Input: part model. Units: mm. Frame: model coordinates. A direction names the side the tool comes from. Coordinates: 2 decimals unless noted, no trailing zeros. Write each loop counter-clockwise with the first axis right and the second up, starting at its lowest first coordinate (ties: lowest second). Pieces come first, ordered by that corner, then holes. Notation, with made-up numbers: (87, 67) - (126, 67) arc R21 ccw to (126, 86) - close; hole circle Ø3 at (-30.75, -23.5). An arc over 180 degrees is marked (long way). One line per question, with ' | ' between items. Start each with the question number.
1) First-contact query: P1, Ø1, axis at x = 2, y = -3.5, coming from the -Z side; P2, Ø1, axis at y = 4, z = -2.5, coming from the -X side; P3, Ø0.8, axis at x = -2.5, y = 3, coming from the -Z side. Flat tips, straight axial feed; report the tip coordinate or a pass-through.
2) Section query A-A on y = 0. Return loops of the section in (x, z), and give its area (3 significant figures).
3) Line query: line 1 (Y direction, x = 0, z = 0.9); line 2 (Z direction, x = -3.5, y = 0.5); line 3 (Y direction, x = -1.75, z = 0.2). Output: solid intervals per line, ascending.
4) Section query B-B on z = 0.65. Return loops of the section in (x, y), and give its area (3 significant figures).
5) Section query C-C on x = 1.5. Return loops of the section in (y, z), and give its area (3 significant figures).
6) Reachability of faces 1 (the flat face through (-2.5, -4.5, -0.5)), 2 (the cylindrical face through (-4.93, 4.94, 1.01)), 3 (the cylindrical face through (-2.565, 3.496, -0.246)) from +Z, -Z, +X, -X, +Y, -Y: full face, straight path, thin tool, end or side. Return the list, or none.
7) Section query D-D on y = 3. Return loops of the section in (x, z).
```python
from build123d import *

# Parameters (mm, degrees)
SKETCH3_W           = 11
SKETCH3_H           = 12.04
BOSS_EXTRUDE1_DEPTH = 2
FILLET1_R           = 2
SKETCH4_R           = 2
CUT_EXTRUDE1_DEPTH  = 2
SKETCH5_R           = 0.5
BOSS_EXTRUDE2_DEPTH = 0.5
SKETCH6_R           = 0.5
BOSS_EXTRUDE3_DEPTH = 4


with BuildPart() as part:
    # Sketch3 → Boss-Extrude1 (new body)
    with BuildSketch(Plane.XY):
        with Locations((0, -0.48)):
            Rectangle(SKETCH3_W, SKETCH3_H)
    extrude(amount=BOSS_EXTRUDE1_DEPTH)

    # Fillet1
    fillet1_edges = [part.edges().sort_by_distance(p)[0] for p in [
        (-5.5, 5.54, 1),
        (5.5, 5.54, 1),
    ]]
    fillet(fillet1_edges, radius=FILLET1_R)

    # Sketch4 → Cut-Extrude1 (cut)
    with BuildSketch(Plane.XY):
        Circle(SKETCH4_R)
    extrude(amount=CUT_EXTRUDE1_DEPTH, mode=Mode.SUBTRACT)

    # Sketch5 → Boss-Extrude2 (add)
    with BuildSketch(Plane.XY):
        with Locations((2.5, 3)):
            Circle(SKETCH5_R)
        with Locations((-2.5, 3)):
            Circle(SKETCH5_R)
        with Locations((2.5, -4.493)):
            Circle(SKETCH5_R)
        with Locations((-2.5, -4.493)):
            Circle(SKETCH5_R)
    extrude(amount=-BOSS_EXTRUDE2_DEPTH)

    # Sketch6 → Boss-Extrude3 (add)
    with BuildSketch(Plane(origin=(0, 0, 0), x_dir=(-1, 0, 0), z_dir=(0, 0, -1))):
        with Locations(Location((0, -6, 0), (0, 0, 270))):
            Circle(SKETCH6_R)
        with Locations(Location((2.5, -6, 0), (0, 0, 270))):
            Circle(SKETCH6_R)
        with Locations(Location((-2.5, -6, 0), (0, 0, 270))):
            Circle(SKETCH6_R)
    extrude(amount=BOSS_EXTRUDE3_DEPTH)


solid = part.part
```
Answer key:
1) P1: z = 0 | P2: through | P3: z = -0.5
2) outline: (-5.5, 0) - (-2, 0) - (-2, 2) - (-5.5, 2) - close; (2, 0) - (5.5, 0) - (5.5, 2) - (2, 2) - close | area: 14.0 mm²
3) line 1: -6.5 to -2, 2 to 5.54 | line 2: 0 to 2 | line 3: -6.5 to -0.97, 0.97 to 5.54
4) outline: (-5.5, -6.5) - (5.5, -6.5) - (5.5, 3.54) arc R2 ccw to (3.5, 5.54) - (-3.5, 5.54) arc R2 ccw to (-5.5, 3.54) - close; hole circle Ø4 at (0, 0) | area: 118 mm²
5) outline: (-6.5, 0) - (-1.32, 0) - (-1.32, 2) - (-6.5, 2) - close; (1.32, 0) - (5.54, 0) - (5.54, 2) - (1.32, 2) - close | area: 18.8 mm²
6) face 1: -Z, +X, -X, +Y | face 2: +Z, -Z, -X, +Y | face 3: -Z
7) outline: (-5.5, 0) - (-3, 0) - (-3, -0.5) - (-2, -0.5) - (-2, 0) - (2, 0) - (2, -0.5) - (3, -0.5) - (3, 0) - (5.5, 0) - (5.5, 2) - (-5.5, 2) - close
